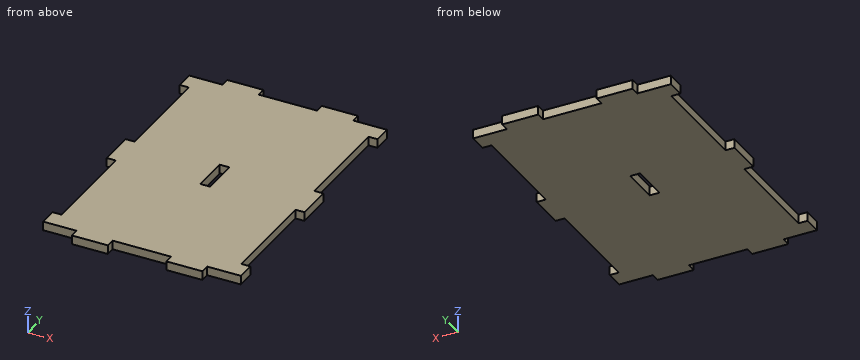
```python
from build123d import *

# Parameters (mm, degrees)
SKETCH2_W           = 5.5
SKETCH2_H           = 20.5
BOSS_EXTRUDE1_DEPTH = 2.5


with BuildPart() as part:
    # Sketch2 → Boss-Extrude1 (new, symmetric)
    with BuildSketch(Plane.XY):
        Polygon((-627.802632857, -77.297008648), (-627.802632857, -72.297008648), (-647.802632857, -72.297008648), (-647.802632857, -77.297008648), (-666.454340614, -77.297008648), (-666.454340614, -87.297008648), (-661.454340614, -87.297008648), (-661.454340614, -144.797008648), (-666.454340614, -144.797008648), (-666.454340614, -164.797008648), (-661.454340614, -164.797008648), (-661.454340614, -222.297008648), (-666.454340614, -222.297008648), (-666.454340614, -232.297008648), (-647.802632857, -232.297008648), (-647.802632857, -237.297008648), (-627.802632857, -237.297008648), (-627.802632857, -232.297008648), (-595.302601942, -232.297008648), (-595.302601942, -237.297008648), (-575.302601942, -237.297008648), (-575.302601942, -232.297008648), (-556.454340614, -232.297008648), (-556.454340614, -222.297008648), (-561.454340614, -222.297008648), (-561.454340614, -164.797008648), (-556.454340614, -164.797008648), (-556.454340614, -144.797008648), (-561.454340614, -144.797008648), (-561.454340614, -87.297008648), (-556.454340614, -87.297008648), (-556.454340614, -77.297008648), (-575.302601942, -77.297008648), (-575.302601942, -72.297008648), (-595.302601942, -72.297008648), (-595.302601942, -77.297008648), align=None)
        with Locations((-611.454340614, -154.797008648)):
            Rectangle(SKETCH2_W, SKETCH2_H, mode=Mode.SUBTRACT)
    extrude(amount=BOSS_EXTRUDE1_DEPTH, both=True)


solid = part.part
```
Can you work these out from the model? Positions are in its coordinate system, mm. Give positions to 0.01 mm unless a question says otherwise; leave off trailing zeros. Write each loop counter-clockwise with the first axis right and the second up, starting at its lowest first coordinate (ties: lowest second). Pieces come first, ordered by that corner, then holes. Notation, with made-up numbers: (70, 41.5) -> (79, 41.5) arc R17 cw to (79, 56.5) -> close; hole circle Ø1 at (41, -17). An arc over 180 degrees is marked (long way). One line per item, written item: value.
Q1. Please list where these lines run through material, in increasing order: line 1 (X direction, y = -159, z = 1.2); line 2 (X direction, y = -114, z = 1.25); line 3 (Y direction, x = -563, z = -0.25). Write a range as [from, to].
Results found:
line 1: x = [-666.45, -614.2], [-608.7, -556.45]
line 2: x = [-661.45, -561.45]
line 3: y = [-232.3, -77.3]
Q2. Imagine slicing it at C-C on y = -192. Please give me the cut outline in (x, z), and give its area (3 significant figures).
Results found:
outline: (-661.45, -2.5) -> (-561.45, -2.5) -> (-561.45, 2.5) -> (-661.45, 2.5) -> close
area: 500 mm^2
Q3. For P1, Ø2.5, axis at x = -613, z = -1, coming from the +Y side; P2, Ø1.5, axis at y = -184, z = -0.5, coming from the -X side; P3, Ø2.5, axis at y = -73.5, z = 1, coming from the -X side, each with a flat end and sliding along its axis, tell me the tip position at first contact or that it passes through.
Results found:
P1: stops at y = -77.3
P2: stops at x = -661.45
P3: stops at x = -647.8
Q4. Imagine slicing it at A-A on y = -162.5. Please give me the cut outline in (x, z).
Results found:
outline: (-666.45, -2.5) -> (-614.2, -2.5) -> (-614.2, 2.5) -> (-666.45, 2.5) -> close; (-608.7, -2.5) -> (-556.45, -2.5) -> (-556.45, 2.5) -> (-608.7, 2.5) -> close
Q5. Imagine slicing it at B-B on x = -658. Please give me the cut outline in (y, z).
Results found:
outline: (-232.3, -2.5) -> (-77.3, -2.5) -> (-77.3, 2.5) -> (-232.3, 2.5) -> close
